from build123d import *

# Parameters (mm, degrees)
F3_R = 10
F4_R = 10


with BuildPart() as f2:
    # F2: sweep along a path in F0
    with BuildLine(Plane.XZ) as f2_path:
        ThreePointArc((-552.9959908712, -429.1799553571), (-307.875, -628.6596729352), (0, -700))
    # F1 (on Right) → F2 (sweep)
    with BuildSketch(Plane.YZ):
        Polygon((0, -717.5), (0, -700), (-50, -700), (-50, -757.5), (-20, -757.5), (-20, -727.5), (-35, -727.5), (-35, -717.5), align=None)
    sweep(path=f2_path.line)

    # F3
    f3_edges = [f2.edges().sort_by_distance(p)[0] for p in [
        (-575.708326, -50, -446.806989),
    ]]
    fillet(f3_edges, radius=F3_R)

    # F4
    f4_edges = [f2.edges().sort_by_distance(p)[0] for p in [
        (0, -50, -728.75),
    ]]
    fillet(f4_edges, radius=F4_R)


solid = f2.part
Read the model definition and answer for the solid it produces. Units are mm, in the model's axes. A direction names the side the tool comes from. Round coordinates to 2 decimals unless told otherwise and drop trailing zeros. Write each loop counter-clockwise with the first axis right and the second up, starting at its lowest first coordinate (ties: lowest second). Pieces come first, ordered by that corner, then holes.
1. Determine the mould class of faces 3 (the face through (-318, -35, -646)), 4 (the face through (-311.877, -25.35, -626.684)), 5 (the face through (-325, -20, -660)) for opening direction X: pulls with the +X half, pulls with the -X half, needs draft (parallel to the pull), parting line crosses it, or undercut.
2. The part is cut by section B-B, the plane z = -585. Determine the outline of the cut face in (x, y), then the cut area to 3 significant figures.
3. Which of the six approach directions +Z, -Z, +X, -X, +Y, -Y give full straight-line access (tool end or side, diameter ignored) to faces 1 (the face through (0, -25, -728)), 2 (the face through (-324.129, -27.605, -651.304))?
4. Straight lines are drawn through the part: L1, parallel to Y at x = -180, z = -712; L2, parallel to X at y = -30.5, z = -650; L3, parallel to Z at x = -229, y = -20.5. For each, find the intervals that lie inside material, in ascending order.
5. The part is cut by section A-A, the plane y = -29. Determine the outline of the cut face in (x, z).
6. The part is cut by section C-C, the plane x = -495.5. Determine the outline of the cut face in (y, z).
7. Given pin 1 Ø1 at (y, z) = (-10, -481.5) entering from -X; pin 2 Ø5 at (y, z) = (-18.5, -670) entering from -X; pin 3 Ø5 at (x, z) = (-319, -691.5) entering from +Y; pin 4 Ø4 at (x, y) = (-224.5, -44.5) entering from +Z, each flat-ended and moving along its own axis, determine where each tip first touches the part or whether it passes through.
Values:
1. face 3: undercut
1. face 4: pulls with the +X half
1. face 5: needs draft
2. outline: (-481.23, -50) - (-384.42, -50) - (-384.42, 0) - (-415.43, 0) - (-415.43, -35) - (-432.47, -35) - (-432.47, -20) - (-481.23, -20) - close
2. area: 3,270 mm2
3. face 1: +Z, -Z, +X, +Y, -Y
3. face 2: +Y
4. L1: y = -50 to -20
4. L2: x = -388.98 to -326.74, -303.82 to -259.81
4. L3: z = -722.06 to -690.52, -679.97 to -661.48
5. outline: (-598.42, -464.43) arc R757.5 ccw to (0, -757.5) - (0, -727.5) arc R727.5 cw to (-574.72, -446.04) - close; (-566.82, -439.91) arc R717.5 ccw to (0, -717.5) - (0, -700) arc R700 cw to (-553, -429.18) - close
6. outline: (-50, -572.96) - (-20, -572.96) - (-20, -532.67) - (-35, -532.67) - (-35, -518.93) - (0, -518.93) - (0, -494.45) - (-50, -494.45) - close
7. pin 1: stops at x = -532.4
7. pin 2: stops at x = -357.19
7. pin 3: passes through
7. pin 4: stops at z = -662.34
